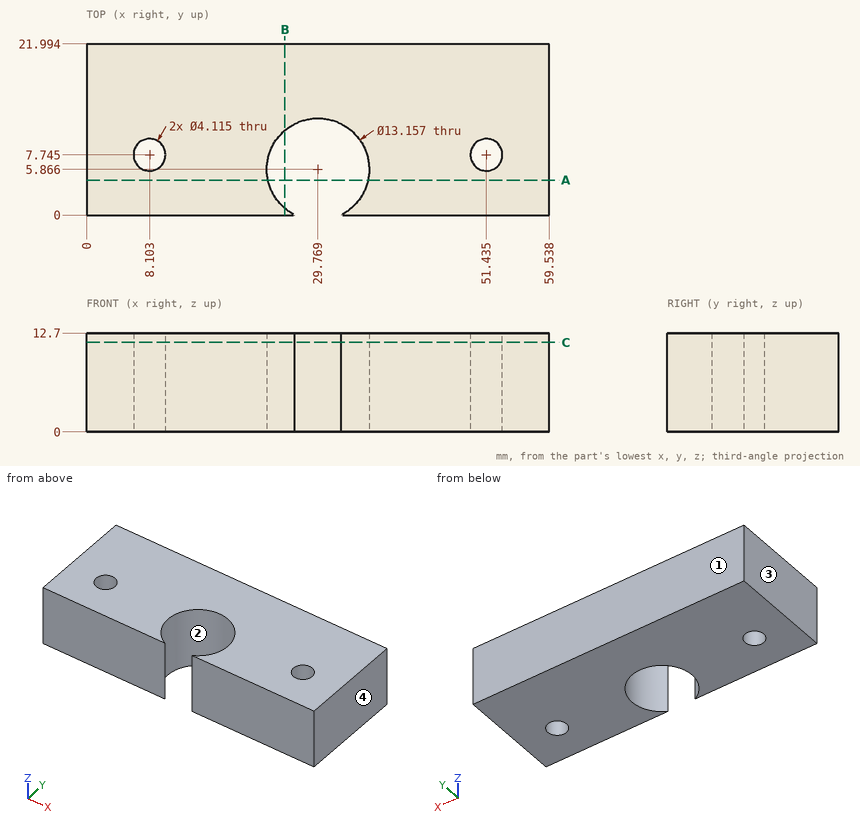
Geometry: see drawing. Coordinates: mm, zero at the bounding-box minimum. Give positions to 0.01 mm unless a question says otherwise; leave off trailing zeros. Order: outer loops, then holes, each group sorted by start corner. A loop starts at its lowest first (then second) coordinate and runs counter-clockwise, first axis right, second up.
Q1. Draft query along X for the marked faces 1, 2, 3 and 4. Return one class per face: +X half, -X half, draft (parallel to the pull), parting line (faces both ways), or undercut.
Checked values:
face 1: draft
face 2: undercut
face 3: -X half
face 4: +X half
Q2. Section A-A on y = 4.5. Output: boundary loops of the cut face in (x, z).
Checked values:
outline: (0, 0) - (23.33, 0) - (23.33, 12.7) - (0, 12.7) - close; (36.2, 0) - (59.54, 0) - (59.54, 12.7) - (36.2, 12.7) - close
Q3. Ray query, probe 1 along X at (y, z) = (5.5, 11.25); probe 2 along X at (y, z) = (11, 8.5) (1 decimal); probe 3 along Y at (x, z) = (24, 11.5) (1 decimal). Return the intervals inside material, ascending.
Checked values:
probe 1: x = 0 to 23.2, 36.34 to 59.54
probe 2: x = 0 to 25.7, 33.9 to 59.5
probe 3: y = 0 to 2.7, 9 to 22
Q4. Section B-B on x = 25.5. Output: boundary loops of the cut face in (y, z), and give its area (3 significant figures).
Checked values:
outline: (0, 0) - (0.86, 0) - (0.86, 12.7) - (0, 12.7) - close; (10.87, 0) - (21.99, 0) - (21.99, 12.7) - (10.87, 12.7) - close
area: 152 mm2
Q5. Section C-C on z = 11.5. Output: boundary loops of the cut face in (x, y) (1 decimal), and give its area (3 significant figures).
Checked values:
outline: (0, 0) - (26.8, 0) arc R6.6 cw (long way) to (32.7, 0) - (59.5, 0) - (59.5, 22) - (0, 22) - close; hole circle Ø4.1 at (8.1, 7.7); hole circle Ø4.1 at (51.4, 7.7)
area: 1,150 mm2
